The model under review builds one solid part; all positions refer to its coordinate system, in mm. A direction names the side the tool comes from. Coordinates: 2 decimals unless noted, no trailing zeros. Write each loop counter-clockwise with the first axis right and the second up, starting at its lowest first coordinate (ties: lowest second). Pieces come first, ordered by that corner, then holes. Notation, with made-up numbers: (-10, 10) -> (41, 10) arc R22 cw to (41, 32) -> close; hole circle Ø3 at (59.25, 46). An arc over 180 degrees is marked (long way). Put each result on its own line as item: value. Start each with the question number.
Autodesk Inventor part; units mm, degrees
ref_plane "YZ Plane" through (0, 0, 0) normal (1, 0, 0) x (0, 1, 0)
ref_plane "XZ Plane" through (0, 0, 0) normal (0, 1, 0) x (-1, 0, 0)
ref_plane "XY Plane" through (0, 0, 0) normal (0, 0, 1) x (1, 0, 0)
sketch "Sketch1" plane through (0, 0, 0) normal (1, 0, 0) x (0, 1, 0)
  line L0 (0, 6) -> (4, 6)
  line L1 (0, -6) -> (4, -6)
  arc A0 (4, -6) -> (4, 6) centre (4, 0) ccw
  line L2 (0, 6) -> (0, 4)
  line L3 (0, 4) -> (-5, 4)
  line L4 (0, -6) -> (0, -4)
  line L5 (0, -4) -> (-5, -4)
  arc A1 (4, -4) -> (4, 4) centre (4, 0) ccw
  line L6 (2, 4) -> (4, 4)
  line L7 (2, -4) -> (4, -4)
  line L8 (2, -4) -> (2, -3)
  line L9 (2, -3) -> (-5, -3)
  line L10 (2, 4) -> (2, 3)
  line L11 (2, 3) -> (-5, 3)
  line L12 (-5, 4) -> (-5, 3)
  line L13 (-5, -3) -> (-5, -4)
  line L14 (-5, 0) -> (10, 0)
  point P0 (0, 0)
  point P1 (8, 0)
  dimension "d0" = 4
  dimension "d1" = 2
  dimension "d2" = 5
  dimension "d3" = 2
  dimension "d4" = 1
  dimension "d5" = 1
revolve "Revolution1" add sketch "Sketch1" angle 360 about axis through (0, -5, 0) along (0, 1, 0) contours A0 L1 L4 L5 L13 L9 L8 L7 A1 L14
properties part number "head"
1. Consider section D-D on x = 0. State the section outline as (y, z) points.
2. Consider section B-B on y = -2.5. State the section outline as (x, z) points, then the cut area to 3 significant figures.
3. Consider section A-A on z = 3.5. State the section outline as (x, y) points, then the cut area to 3 significant figures.
4. The part is to be moulded in two halves that separate along Z. For faces 1 (the flat face through (3.92, 0, 1.42)), 2 (the cylindrical face through (3.905, 3.014, 0.867)), 3 (the cylindrical face through (0, 2, 6)), say which applies: released by +Z, released by -Z, zero draft, split by the parting line, or undercut.
5. Wall thickness on line 1 (X direction, y = -0.75, z = 0); line 2 (Z direction, x = 0, y = 3.4): over which ranges is each line inside the solid? List them lowest first. Write a range as from..to.
6. Insertion check: P1, Ø3, axis at y = 5, z = 4.5, coming from the +X side; P2, Ø3, axis at y = -2, z = -3.5, coming from the +X side; P3, Ø2.5, axis at x = 1.5, z = 0.5, coming from the +Y side; P4, Ø4, axis at y = 2, z = -0.5, coming from the -X side. Each pin has a flat end and moves straight along its axis. Give the tip position at first contact, or say it passes through.
7. Consider section C-C on z = 0. State the section outline as (x, y) points, then the cut area to 3 significant figures.
8. Tool access review of faces 4 (the cylindrical face through (-3.905, -2.535, 0.867)), 5 (the flat face through (-3, 2, -1)), 6 (the flat face through (-3, -5, -1)): name each direction out of +Z, -Z, +X, -X, +Y, -Y from which nothing blocks a thin tool from reaching the whole face with its end or side.
Output values:
1. outline: (-5, -4) -> (0, -4) -> (0, -6) -> (4, -6) arc R6 ccw to (4, 6) -> (0, 6) -> (0, 4) -> (-5, 4) -> (-5, 3) -> (2, 3) -> (2, 4) -> (4, 4) arc R4 cw to (4, -4) -> (2, -4) -> (2, -3) -> (-5, -3) -> close
2. outline: circle Ø8 at (0, 0); hole circle Ø6 at (0, 0)
2. area: 22.0 mm^2
3. outline: (-4.87, 0) -> (-1.94, 0) -> (-1.94, -5) -> (1.94, -5) -> (1.94, 0) -> (4.87, 0) -> (4.87, 4) arc R4.87 ccw to (-4.87, 4) -> close; hole (-1.94, 2) -> (1.94, 2) -> (1.94, 4) arc R1.94 ccw to (-1.94, 4) -> close
3. area: 82.0 mm^2
4. face 1: zero draft
4. face 2: undercut
4. face 3: split by the parting line
5. line 1: x = -4..-3, 3..4
5. line 2: z = -6..-4, 4..6
6. P1: stops at x = 5.13
6. P2: stops at x = 3.46
6. P3: stops at y = 9.99
6. P4: stops at x = -6
7. outline: (-6, 0) -> (-4, 0) -> (-4, -5) -> (-3, -5) -> (-3, 2) -> (-4, 2) -> (-4, 4) arc R4 cw to (4, 4) -> (4, 2) -> (3, 2) -> (3, -5) -> (4, -5) -> (4, 0) -> (6, 0) -> (6, 4) arc R6 ccw to (-6, 4) -> close
7. area: 61.4 mm^2
8. face 4: -Y
8. face 5: none
8. face 6: +Z, -Z, +X, -X, -Y
